```python
from build123d import *

# Parameters (mm, degrees)
F0_W     = 127
F0_H     = 127
F1_DEPTH = 63.5
F3_DEPTH = 101.6


with BuildPart() as f1:
    # F0 (on Top) → F1 (new body, symmetric)
    with BuildSketch(Plane.XY):
        with Locations((-0.111125, -0.834118)):
            Rectangle(F0_W, F0_H)
    extrude(amount=F1_DEPTH, both=True)

    # F2 (on face) → F3 (cut)
    with BuildSketch(Plane.XY.offset(63.5)):
        Polygon((63.388875, -64.334118), (63.388875, -13.534118), (12.588875, -64.334118), align=None)
        Polygon((-12.811125, 62.665882), (-63.611125, 62.665882), (-63.611125, 11.865882), align=None)
    extrude(amount=-F3_DEPTH, mode=Mode.SUBTRACT)


solid = f1.part
```
The listing builds one solid part. Answer for the finished solid, in the listing's coordinates (mm). A direction names the side the tool comes from. Coordinates: 2 decimals unless noted, no trailing zeros. Write each loop counter-clockwise with the first axis right and the second up, starting at its lowest first coordinate (ties: lowest second). Pieces come first, ordered by that corner, then holes.
Q1. Section B-B, the plane y = 45 is taken. Write down the section's boundary in (x, z).
Returned:
outline: (-63.61, -63.5) - (63.39, -63.5) - (63.39, 63.5) - (-30.48, 63.5) - (-30.48, -38.1) - (-63.61, -38.1) - close
Q2. Given P1, Ø8, axis at x = -24.5, z = 32.5, coming from the +Y side; P2, Ø12, axis at x = -48.5, y = 39.5, coming from the +Z side, each flat-ended and moving along its own axis, determine where each tip first touches the part or whether it passes through.
Returned:
P1: stops at y = 54.98
P2: stops at z = -38.1
Q3. Find the intervals of material crossed by line 1 along Y through (x, z) = (17, 24.5); line 2 along X through (y, z) = (57.5, 24.5); line 3 along Y through (x, z) = (17.5, 45), in increasing order.
Returned:
line 1: y = -59.92 to 62.67
line 2: x = -17.98 to 63.39
line 3: y = -59.42 to 62.67
Q4. Section A-A, the plane z = 13.5 is taken. Write down the section's boundary in (x, y), then the cut area to 3 significant figures.
Returned:
outline: (-63.61, -64.33) - (12.59, -64.33) - (63.39, -13.53) - (63.39, 62.67) - (-12.81, 62.67) - (-63.61, 11.87) - close
area: 13,500 mm2
Q5. Which of the six approach directions +Z, -Z, +X, -X, +Y, -Y give full straight-line access (tool end or side, diameter ignored) to faces 1 (the flat face through (38.344, -38.579, 13.411)), 2 (the flat face through (-44, 43, -38.1)), 3 (the flat face through (-1, 0, -63.5))?
Returned:
face 1: +Z, +X, -Y
face 2: +Z, -X, +Y
face 3: -Z, +X, -X, +Y, -Y
